Print and shaded views of the part. All mm, measured from the part's lowest x, y and z. Round coordinates to 2 decimals unless told otherwise and drop trailing zeros. Loops run counter-clockwise (first coordinate to the right, second up) from the corner with the lowest first, then second, coordinate; pieces in that order, holes last. Notation, with made-up numbers: (36, 89) -> (55, 89) arc R27 cw to (55, 114) -> close; hole circle Ø9 at (28.5, 7.25). An arc over 180 degrees is marked (long way). Answer as CSV lines item,"result".
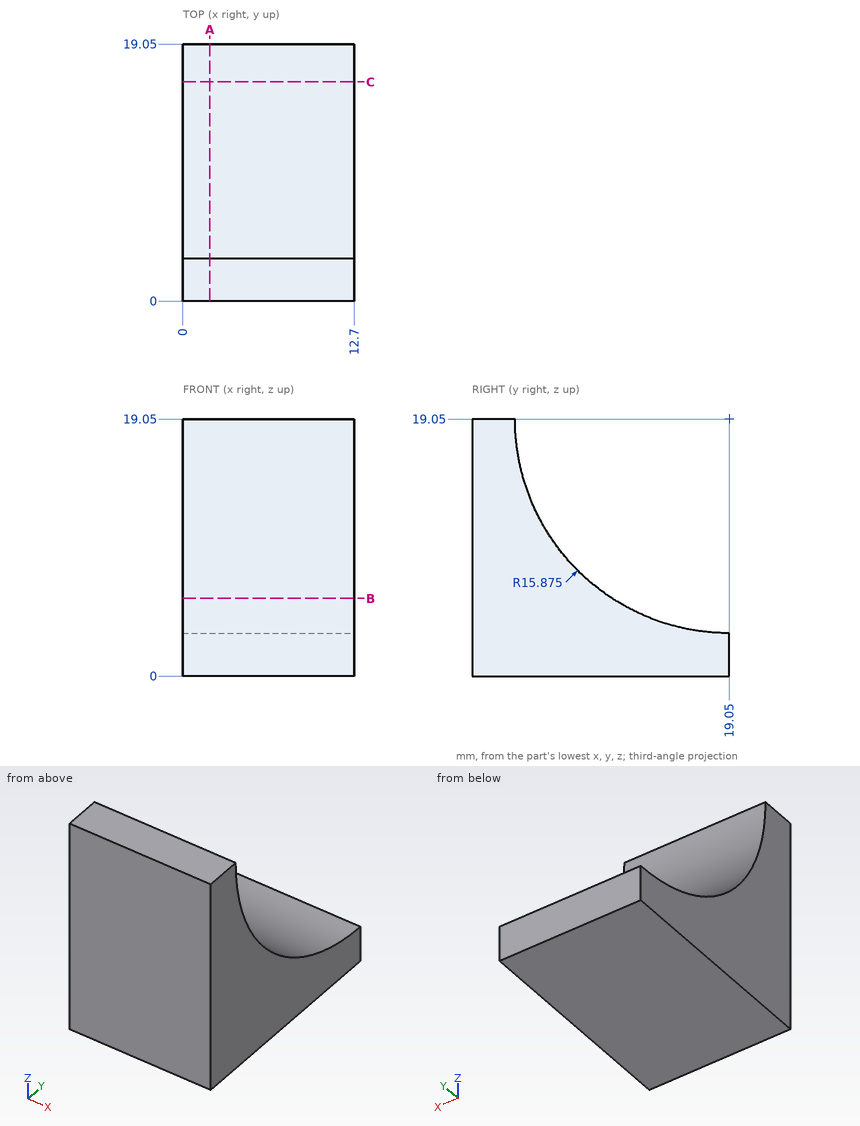
Q1. Drop a flat-ended pin along its axis: P1, Ø1.5, axis at x = 3.5, z = 11.5, coming from the +Y side. Give the stop position or say it passes through.
Geometry results:
P1,"y = 5.52"
Q2. Saw through at C-C, the plane y = 16.25. Write the cut outline in (x, z).
Geometry results:
outline,"(0, 0) -> (12.7, 0) -> (12.7, 3.42) -> (0, 3.42) -> close"
Q3. Saw through at B-B, the plane z = 5.75. Write the cut outline in (x, y), then the cut area to 3 significant figures.
Geometry results:
outline,"(0, 0) -> (12.7, 0) -> (12.7, 10.38) -> (0, 10.38) -> close"
area,"132 mm2"
Q4. Saw through at A-A, the plane x = 2. Write the cut outline in (y, z) (3 decimals).
Geometry results:
outline,"(0, 0) -> (19.05, 0) -> (19.05, 3.175) arc R15.875 cw to (3.175, 19.05) -> (0, 19.05) -> close"
Q5. Drill centre lines: line 1 along Z through (x, y) = (10.5, 4.5); line 2 along Z through (x, y) = (10.75, 7.5); line 3 along Y through (x, z) = (2.75, 10.5). Where is each one in solid material? Low to high.
Geometry results:
line 1,"0 to 12.7"
line 2,"0 to 8.16"
line 3,"0 to 5.67"
